```python
from build123d import *

# Parameters (mm, degrees)
SKETCH1_R           = 2
BOSS_EXTRUDE1_DEPTH = 4
SKETCH2_W           = 8
SKETCH2_H           = 1
CUT_EXTRUDE1_DEPTH  = 32
SKETCH2_2_W         = 8
SKETCH2_2_H         = 1
CUT_EXTRUDE2_DEPTH  = 35


with BuildPart() as part:
    # Sketch1 → Boss-Extrude1 (new body)
    with BuildSketch(Plane(origin=(0, 0, 0), x_dir=(1, 0, 0), z_dir=(0, 1, 0))):
        with BuildLine():
            Line((24, -6), (-24, -6))
            ThreePointArc((-24, -6), (-30, 0), (-24, 6))
            Line((-24, 6), (24, 6))
            ThreePointArc((24, 6), (30, 0), (24, -6))
        make_face()
        with Locations(Location((-24, 0, 0), (0, 0, 270))):
            Circle(SKETCH1_R, mode=Mode.SUBTRACT)
        with Locations(Location((-16, 0, 0), (0, 0, 270))):
            Circle(SKETCH1_R, mode=Mode.SUBTRACT)
        with Locations(Location((-8, 0, 0), (0, 0, 270))):
            Circle(SKETCH1_R, mode=Mode.SUBTRACT)
        with Locations(Location((0, 0, 0), (0, 0, 270))):
            Circle(SKETCH1_R, mode=Mode.SUBTRACT)
        with Locations(Location((8, 0, 0), (0, 0, 90))):
            Circle(SKETCH1_R, mode=Mode.SUBTRACT)
        with Locations(Location((16, 0, 0), (0, 0, 90))):
            Circle(SKETCH1_R, mode=Mode.SUBTRACT)
        with Locations(Location((24, 0, 0), (0, 0, 90))):
            Circle(SKETCH1_R, mode=Mode.SUBTRACT)
    extrude(amount=BOSS_EXTRUDE1_DEPTH)

    # Sketch2 → Cut-Extrude1 (cut)
    with BuildSketch(Plane(origin=(0, 0, 0), x_dir=(0, 0, -1), z_dir=(1, 0, 0))):
        with Locations((0, 3.5)):
            Rectangle(SKETCH2_W, SKETCH2_H)
    extrude(amount=-CUT_EXTRUDE1_DEPTH, mode=Mode.SUBTRACT)

    # Sketch2_2 → Cut-Extrude2 (cut)
    with BuildSketch(Plane(origin=(0, 0, 0), x_dir=(0, 0, -1), z_dir=(1, 0, 0))):
        with Locations((0, 3.5)):
            Rectangle(SKETCH2_2_W, SKETCH2_2_H)
    extrude(amount=CUT_EXTRUDE2_DEPTH, mode=Mode.SUBTRACT)


solid = part.part
```
Design review of the part built by this model. Coordinates are the model's own, in mm. A direction names the side the tool comes from. Round coordinates to 2 decimals unless told otherwise and drop trailing zeros. Write each loop counter-clockwise with the first axis right and the second up, starting at its lowest first coordinate (ties: lowest second). Pieces come first, ordered by that corner, then holes.
Item 1: We need section A-A on z = 0. State how many separate pieces and enclosed holes the cut face has, and give its area (3 significant figures).
Item 2: We need section B-B on x = -8. Write out the cut boundary in (y, z), and give its area (3 significant figures).
Item 3: Clearance check with flat-ended pins moving along their axes: pin 1 Ø1.5 at (y, z) = (3.5, 0) entering from -X; pin 2 Ø1 at (y, z) = (2.5, 2.5) entering from -X; pin 3 Ø3 at (x, z) = (16, 0) entering from -Y; pin 4 Ø6.5 at (x, z) = (8, 0) entering from +Y. State where each tip first meets the part, or that it passes through.
Item 4: For faces 4 (the flat face through (0, 3, 3)), 5 (the cylindrical face through (6, 1, 0)), list the 3-axis set-ups (+Z, -Z, +X, -X, +Y, -Y) from which the entire face can be reached by the end or side of a thin tool; tool diameter is ignored.
Item 5: We need section C-C on x = 10.5. Write out the cut boundary in (y, z), and give its area (3 significant figures).
Item 6: The part is to be moulded in two halves that separate along X. For faces 1 (the cylindrical face through (-30, 2, 0)), 2 (the cylindrical face through (-2, 1, 0)), 3 (the flat face through (0, 0, -3)), say which applies: +X half, -X half, draft (parallel to the pull), parting line (faces both ways), or undercut.
Item 7: For probe 1 along Z at (x, y) = (16, 1.95); probe 2 along Y at (x, z) = (20.5, -0.5); probe 3 along Z at (x, y) = (1, 3.35), list the stretches that pass through material, from the lowest coordinate up.
Item 8: We need section D-D on y = 2.2. Write out the cut boundary in (x, z).
Returned:
1. separate pieces: 8
1. enclosed holes: 0
1. area: 96.0 mm2
2. outline: (0, -6) - (4, -6) - (4, -4) - (3, -4) - (3, -2) - (0, -2) - close; (0, 2) - (3, 2) - (3, 4) - (4, 4) - (4, 6) - (0, 6) - close
2. area: 28.0 mm2
3. pin 1: stops at x = -30
3. pin 2: stops at x = -29.66
3. pin 3: passes through
3. pin 4: stops at y = 3
4. face 4: +X, -X, +Y
4. face 5: +Y, -Y
5. outline: (0, -6) - (4, -6) - (4, -4) - (3, -4) - (3, 4) - (4, 4) - (4, 6) - (0, 6) - close
5. area: 40.0 mm2
6. face 1: -X half
6. face 2: undercut
6. face 3: draft
7. probe 1: z = -6 to -2, 2 to 6
7. probe 2: y = 0 to 3
7. probe 3: z = -6 to -4, 4 to 6
8. outline: (-24, -6) - (24, -6) arc R6 ccw to (24, 6) - (-24, 6) arc R6 ccw to start; hole circle Ø4 at (-24, 0); hole circle Ø4 at (-16, 0); hole circle Ø4 at (-8, 0); hole circle Ø4 at (0, 0); hole circle Ø4 at (8, 0); hole circle Ø4 at (16, 0); hole circle Ø4 at (24, 0)
